from build123d import *

# Parameters (mm, degrees)
SKETCH1_R                = 19
BOSS_EXTRUDE1_DEPTH      = 3.5
SKETCH2_R                = 30
SKETCH2_R_2              = 19
SKETCH2_R_3              = 2.8
BOSS_EXTRUDE2_DEPTH      = 5
BOSS_EXTRUDE3_DEPTH      = 2
BOSS_EXTRUDE3_DEPTH_BACK = 5
SKETCH4_R                = 2.9
SKETCH5_R                = 5
BOSS_EXTRUDE4_DEPTH      = 3
CUT_EXTRUDE1_START       = -10
SKETCH3_R                = 19
CUT_EXTRUDE1_DEPTH       = 10
CUT_EXTRUDE3_START       = -13
CUT_EXTRUDE3_DEPTH       = 13
FILLET1_R                = 10
FILLET2_R                = 5
CUT_EXTRUDE4_START       = -3
SKETCH8_R                = 4
SKETCH8_R_2              = 19
CUT_EXTRUDE4_DEPTH       = 3
FILLET3_R                = 1


with BuildPart() as part:
    # Sketch1 → Boss-Extrude1 (new body)
    with BuildSketch(Plane(origin=(0, 0, 0), x_dir=(1, 0, 0), z_dir=(0, 1, 0))):
        with Locations(Location((0, 0, 0), (0, 0, 270))):
            Circle(SKETCH1_R)
    extrude(amount=BOSS_EXTRUDE1_DEPTH)

    # Sketch2 → Boss-Extrude2 (add)
    with BuildSketch(Plane(origin=(0, 0, 0), x_dir=(1, 0, 0), z_dir=(0, 1, 0))):
        with Locations(Location((0, 0, 0), (0, 0, 270))):
            Circle(SKETCH2_R)
        with Locations(Location((0, 0, 0), (0, 0, 270))):
            Circle(SKETCH2_R_2, mode=Mode.SUBTRACT)
        with Locations(Location((0, 25, 0), (0, 0, 270))):
            Circle(SKETCH2_R_3, mode=Mode.SUBTRACT)
        with Locations(Location((21.650635095, -12.5, 0), (0, 0, 270))):
            Circle(SKETCH2_R_3, mode=Mode.SUBTRACT)
        with Locations(Location((-21.650635095, -12.5, 0), (0, 0, 270))):
            Circle(SKETCH2_R_3, mode=Mode.SUBTRACT)
    extrude(amount=BOSS_EXTRUDE2_DEPTH)

    # Sketch4 → Boss-Extrude3 (add, two sides: drawn at the far end of the back side and taken through both)
    with BuildSketch(Plane.XZ.offset(-BOSS_EXTRUDE3_DEPTH_BACK)):
        with Locations(Location((-21.650635095, 12.5, 0), (0, 0, 270))):
            Circle(SKETCH4_R)
        with Locations(Location((21.650635095, 12.5, 0), (0, 0, 270))):
            Circle(SKETCH4_R)
        with Locations(Location((0, -25, 0), (0, 0, 270))):
            Circle(SKETCH4_R)
    extrude(amount=BOSS_EXTRUDE3_DEPTH + BOSS_EXTRUDE3_DEPTH_BACK)

    # Sketch5 → Boss-Extrude4 (add)
    with BuildSketch(Plane(origin=(0, 5, 0), x_dir=(1, 0, 0), z_dir=(0, 1, 0))):
        with Locations((-26.103110985, -14.7860609)):
            Circle(SKETCH5_R)
        with Locations((0.246451131, 29.99898768)):
            Circle(SKETCH5_R)
        with Locations((25.856659853, -15.212926781)):
            Circle(SKETCH5_R)
    extrude(amount=-BOSS_EXTRUDE4_DEPTH)

    # Sketch3 → Cut-Extrude1 (cut)
    with BuildSketch(Plane(origin=(0, 3.5, 0), x_dir=(1, 0, 0), z_dir=(0, 1, 0)).offset(CUT_EXTRUDE1_START)):
        with Locations(Location((0, 0, 0), (0, 0, 270))):
            Circle(SKETCH3_R)
    extrude(amount=CUT_EXTRUDE1_DEPTH, mode=Mode.SUBTRACT)

    # Sketch7 → Cut-Extrude3 (cut)
    with BuildSketch(Plane(origin=(0, 5, 0), x_dir=(1, 0, 0), z_dir=(0, 1, 0)).offset(CUT_EXTRUDE3_START)):
        with BuildLine():
            ThreePointArc((-29.54423259, -5.20944533), (-25.980762114, 15), (-10.2606043, 28.190778624))
            Line((-10.2606043, 28.190778624), (-13.773984089, 37.84371026))
            Line((-13.773984089, 37.84371026), (-43.939319858, -7.747687605))
            Line((-43.939319858, -7.747687605), (-29.54423259, -5.20944533))
        make_face()
        with BuildLine():
            ThreePointArc((-26.13264562, -4.6078905), (-22.980662881, 13.267891901), (-9.075772579, 24.935480225))
            Line((-9.075772579, 24.935480225), (-10.2606043, 28.190778624))
            ThreePointArc((-10.2606043, 28.190778624), (-25.980762114, 15), (-29.54423259, -5.20944533))
            Line((-29.54423259, -5.20944533), (-26.13264562, -4.6078905))
        make_face()
        with BuildLine():
            Line((15.259965643, 41.926411025), (10.2606043, 28.190778624))
            ThreePointArc((10.2606043, 28.190778624), (25.980762114, 15), (29.54423259, -5.20944533))
            Line((29.54423259, -5.20944533), (39.660606503, -6.993234998))
            Line((39.660606503, -6.993234998), (15.259965643, 41.926411025))
        make_face()
        with BuildLine():
            Line((10.2606043, 28.190778624), (9.075772579, 24.935480225))
            ThreePointArc((9.075772579, 24.935480225), (21.736841548, 15.220300308), (26.535783801, 0))
            ThreePointArc((26.535783801, 0), (26.434807132, -2.312745947), (26.13264562, -4.6078905))
            Line((26.13264562, -4.6078905), (29.54423259, -5.20944533))
            ThreePointArc((29.54423259, -5.20944533), (25.980762114, 15), (10.2606043, 28.190778624))
        make_face()
        with BuildLine():
            Line((28.679354216, -34.17872342), (19.283628291, -22.981333294))
            ThreePointArc((19.283628291, -22.981333294), (0, -30), (-19.283628291, -22.981333294))
            Line((-19.283628291, -22.981333294), (-25.886622414, -30.850475262))
            Line((-25.886622414, -30.850475262), (28.679354216, -34.17872342))
        make_face()
        with BuildLine():
            Line((19.283628291, -22.981333294), (17.056873041, -20.327589725))
            ThreePointArc((17.056873041, -20.327589725), (0, -26.535783801), (-17.056873041, -20.327589725))
            Line((-17.056873041, -20.327589725), (-19.283628291, -22.981333294))
            ThreePointArc((-19.283628291, -22.981333294), (0, -30), (19.283628291, -22.981333294))
        make_face()
    extrude(amount=CUT_EXTRUDE3_DEPTH, mode=Mode.SUBTRACT)

    # Fillet1
    # the kernel refuses this fillet: 10 mm, written as the material it adds along each edge
    with BuildSketch(Plane(origin=(-26.13264562, 0, 4.6078905), x_dir=(-0.9848077530122318, 0, 0.17364817766679624), z_dir=(0, 1, 0)), Plane(origin=(17.056873041, 0, 20.327589725), x_dir=(0.6427876096865569, 0, 0.7660444431189634), z_dir=(0, 1, 0)), Plane(origin=(9.075772579, 0, -24.935480225), x_dir=(0.34202014332561265, 0, -0.9396926207859289), z_dir=(0, 1, 0))) as fillet1_piece_1:
        with BuildLine():
            CenterArc((9.045274498, -8.297697769), FILLET1_R, 123.92490422, 42.948020906)
            Line((-0.693413056, -6.026582466), (-0.888186807, -5.98116016))
            ThreePointArc((-0.888186807, -5.98116016), (-0.372612378, -3.01031053), (-0.2, 0))
            Line((-0.2, 0), (0, 0.2))
            ThreePointArc((0, 0.2), (1.732108099, 0.2), (3.352595033, 0.165953955))
            Line((3.352595033, 0.165953955), (3.464216199, 0))
        make_face()
    extrude(amount=5)
    with BuildSketch(Plane(origin=(-17.056873041, 0, 20.327589725), x_dir=(0.8344973728156843, 0, 0.551011918894429), z_dir=(0, 1, 0)), Plane(origin=(26.13264562, 0, 4.6078905), x_dir=(0.059941633142754296, 0, -0.99820188369697), z_dir=(0, 1, 0)), Plane(origin=(-9.075772579, 0, -24.935480225), x_dir=(-0.8944390059584274, 0, 0.44718996480254386), z_dir=(0, 1, 0))) as fillet1_piece_2:
        with BuildLine():
            CenterArc((7.20939257, -9.934457095), FILLET1_R, 96.563537437, 42.948020906)
            Line((-0.39597707, -3.441510719), (-0.548084463, -3.311651792))
            ThreePointArc((-0.548084463, -3.311651792), (-0.396677677, -1.697894369), (-0.198689142, 0.022860991))
            Line((-0.198689142, 0.022860991), (0.022860991, 0.198689142))
            ThreePointArc((0.022860991, 0.198689142), (3.03317152, 0.026076764), (6.04348205, 0.198689142))
            Line((6.04348205, 0.198689142), (6.06634304, 0))
        make_face()
    extrude(amount=5)

    # Fillet2
    fillet2_edges = [part.edges().sort_by_distance(p)[0] for p in [
        (-10.2606043, 2.5, -28.190778624),
        (-29.54423259, 2.5, 5.20944533),
        (-19.283628291, 2.5, 22.981333294),
        (19.283628291, 2.5, 22.981333294),
        (29.54423259, 2.5, 5.20944533),
        (10.2606043, 2.5, -28.190778624),
    ]]
    fillet(fillet2_edges, radius=FILLET2_R)

    # Sketch8 → Cut-Extrude4 (cut)
    with BuildSketch(Plane(origin=(0, 5, 0), x_dir=(1, 0, 0), z_dir=(0, 1, 0)).offset(CUT_EXTRUDE4_START)):
        with Locations((-16.524893724, 9.376987118)):
            Circle(SKETCH8_R)
        with Locations(Location((0, 0, 0), (0, 0, 42.512080704))):
            Circle(SKETCH8_R_2)
        with Locations((16.383155917, 9.622484201)):
            Circle(SKETCH8_R)
        with Locations((0.141737807, -18.999471319)):
            Circle(SKETCH8_R)
    extrude(amount=CUT_EXTRUDE4_DEPTH, mode=Mode.SUBTRACT)

    # Fillet3
    # the kernel refuses this fillet: 1 mm, written as the material it takes off along each edge
    with BuildSketch(Plane(origin=(-18.121826323, 6.950278825, -5.709589366), x_dir=(-0.28086097725665193, 0, 0.9597484625955065), z_dir=(0, -1, 0)), Plane(origin=(14.005562597, 6.950278825, -12.839167276), x_dir=(-0.6907360612225409, 0, -0.7231069725336425), z_dir=(0, -1, 0))) as fillet3_piece_1:
        with BuildLine():
            CenterArc((0.800640781, 0.999789253), FILLET3_R, 197.486602821, 71.337075115)
            ThreePointArc((-0.153146456, 0.699306464), (-0.060897436, 0.353086193), (0, 0))
            ThreePointArc((0, 0), (0.390055765, 0.004004198), (0.78011153, 0))
        make_face()
    extrude(amount=4.950278825, mode=Mode.SUBTRACT)
    with BuildSketch(Plane(origin=(-14.195555863, 6.950278825, -12.628784333), x_dir=(-0.8617980531882996, 0, -0.5072515308216002), z_dir=(0, -1, 0)), Plane(origin=(18.034625983, 6.950278825, -5.979319831), x_dir=(0.8701917383942803, 0, -0.49271324158209956), z_dir=(0, -1, 0))) as fillet3_piece_2:
        with BuildLine():
            CenterArc((0.805364366, 0.995988176), FILLET3_R, 193.528948716, 71.337075115)
            ThreePointArc((-0.166887482, 0.762051552), (-0.079532242, 0.381882385), (0, 0))
            ThreePointArc((0, 0), (0.357939718, 0.016047295), (0.715879437, 0))
        make_face()
    extrude(amount=4.950278825, mode=Mode.SUBTRACT)
    with BuildSketch(Plane(origin=(4.116263726, 6.950278825, 18.548756641), x_dir=(0.023311579398747933, 0, 0.9997282482084497), z_dir=(0, -1, 0))) as fillet3_piece_3:
        with BuildLine():
            CenterArc((0.805364366, -0.995988176), FILLET3_R, 95.133976169, 71.337075115)
            ThreePointArc((-0.166887482, -0.762051552), (-0.079532242, -0.381882385), (0, 0))
            ThreePointArc((0, 0), (0.357939718, -0.016047295), (0.715879437, 0))
        make_face()
    extrude(amount=4.950278825, mode=Mode.SUBTRACT)
    with BuildSketch(Plane(origin=(-3.83907012, 6.950278825, 18.608104165), x_dir=(-0.9750194381231715, 0, -0.22211955177780904), z_dir=(0, -1, 0))) as fillet3_piece_4:
        with BuildLine():
            CenterArc((0.800640781, -0.999789253), FILLET3_R, 91.176322064, 71.337075115)
            ThreePointArc((-0.153146456, -0.699306464), (-0.060897436, -0.353086193), (0, 0))
            ThreePointArc((0, 0), (0.390055765, -0.004004198), (0.78011153, 0))
        make_face()
    extrude(amount=4.950278825, mode=Mode.SUBTRACT)


solid = part.part
The model under review builds one solid part; all positions refer to its coordinate system, in mm. A direction names the side the tool comes from. Give positions to 0.01 mm unless a question says otherwise; leave off trailing zeros. Order: outer loops, then holes, each group sorted by start corner. A loop starts at its lowest first (then second) coordinate and runs counter-clockwise, first axis right, second up. Notation, with made-up numbers: M -36,87.5 L -1,87.5 A24 cw -1,100.5 Z; hole C 79,38 d11. An arc over 180 degrees is marked long. Answer in a Markdown table with one row per item. Add a question column.
1. For pin 1 Ø2.5 at (x, z) = (-28, 14.5) entering from -Y; pin 2 Ø4.5 at (x, z) = (0, -32) entering from -Y; pin 3 Ø1 at (x, z) = (-21.5, -19) entering from +Y; pin 4 Ø2 at (x, z) = (17, -9.5) entering from +Y, all flat-tipped, find the tip position at first contact; note any pin that passes through.
2. Add section C-C on z = -11. State the section outline as (x, y) points.
3. Add section D-D on y = -1. State the section outline as (x, z) points, plus the area to 3 significant figures.
4. Add section B-B on x = 1.5. State the section outline as (y, z) points.
5. To check wall thickness, follow line 1 along Z through (x, y) = (0, 3.05); line 2 along Y through (x, z) = (-14.5, -21); line 3 along Z through (x, y) = (6.5, 4.75). State the ranges of each line that lie inside material, in increasing order.
6. Add section A-A on z = 0. State the section outline as (x, y) points.
7. Mouldability with a two-part tool opening along Z and no side actions: class faces 1 (the cylindrical face through (14.62, 2.46, 22.77)), 2 (the flat face through (0, -2, -25)), 3 (the cylindrical face through (25.93, 1.35, 15.09)) as released by +Z, released by -Z, zero draft, split by the parting line, or undercut.
8. Machinability: for faces 4 (the cylindrical face through (21.778, -0.986, 15.397)), 5 (the cylindrical face through (0.1, 3.5, 23)), 6 (the flat face through (-28, 2, 16)), 7 (the flat face through (-22, -2, 13)), which of the approach directions +Z, -Z, +X, -X, +Y, -Y give a long, thin tool a straight path to every point of the face, cutting with its end or side? Answer none if there is none.
The answers:
| question | item | result |
|---|---|---|
| 1 | pin 1 | y = 2 |
| 1 | pin 2 | y = 0 |
| 1 | pin 3 | through |
| 1 | pin 4 | y = 2 |
| 2 | outline | M -24.15,0 L -15.49,0 L -15.49,2 L -20.18,2 L -20.18,5 L -24.15,5 Z; M 15.49,0 L 24.15,0 L 24.15,5 L 20.14,5 L 20.14,2 L 15.49,2 Z |
| 3 | outline | C -21.65,12.5 d5.8; C 0,-25 d5.8; C 21.65,12.5 d5.8 |
| 3 | area | 79.3 mm2 |
| 4 | outline | M -2,-27.48 L 0,-27.48 L 0,-29.96 L 2,-29.96 L 2,-34.84 L 5,-34.84 L 5,-18.94 L 0,-18.94 L 0,-22.52 L -2,-22.52 Z; M 0,18.94 L 2,18.94 L 2,22.76 L 5,22.76 L 5,26.49 L 0,26.49 Z |
| 5 | line 1 | -34.99 to -19, 23 to 26.54 |
| 5 | line 2 | 0 to 5 |
| 5 | line 3 | -29.29 to -17.85, 17.85 to 25.73 |
| 6 | outline | M -26.68,0 L -19,0 L -19,5 L -26.68,5 Z; M 19,0 L 26.68,0 L 26.68,5 L 19,5 Z |
| 7 | face 1 | released by +Z |
| 7 | face 2 | zero draft |
| 7 | face 3 | undercut |
| 8 | face 4 | -Y |
| 8 | face 5 | +Y |
| 8 | face 6 | +Z, -X, -Y |
| 8 | face 7 | +Z, -Z, +X, -X, -Y |
